Geometry check sheet. Reference: the model listing, model coordinates, mm. A direction names the side the tool comes from. Coordinates: 2 decimals unless noted, no trailing zeros. Write each loop counter-clockwise with the first axis right and the second up, starting at its lowest first coordinate (ties: lowest second). Pieces come first, ordered by that corner, then holes. Notation, with made-up numbers: M 23,-8 L 48,-8 A21 cw 48,30 Z; hole C 58.25,38.25 d1. An arc over 180 degrees is marked long. Write each question's results on one line, items separated by ' | '.
```python
from build123d import *

# Parameters (mm, degrees)
F0_R          = 3.75
F1_DEPTH      = 25
F2_W          = 29.9994934789
F2_H          = 9
F3_DEPTH      = 52
F5_DEPTH      = 25
F8_DEPTH      = 3.5
F8_DEPTH_BACK = 3.5


with BuildPart() as f1:
    # F0 (on Top) → F1 (new body)
    with BuildSketch(Plane.XY):
        with BuildLine():
            Line((0, 18.1232695296), (0, 0))
            Line((0, 0), (29.9994934789, 0))
            Line((29.9994934789, 0), (29.9994934789, 18))
            ThreePointArc((29.9994934789, 18), (15.061128764, 32.9998733692), (0, 18.1232695296))
        make_face()
        with Locations((14.9994934789, 18)):
            Circle(F0_R, mode=Mode.SUBTRACT)
    extrude(amount=F1_DEPTH)

    # F2 (on face) → F3 (join)
    with BuildSketch(Plane.XZ):
        with Locations((14.9997467394, 4.5)):
            Rectangle(F2_W, F2_H)
    extrude(amount=F3_DEPTH)

    # F4 (on face) → F5 (cut)
    with BuildSketch(Plane.XY.offset(9)):
        Polygon((20.9994934789, -52), (29.9994934789, -52), (29.9994934789, -43), align=None)
        Polygon((0, -43), (0, -52), (9, -52), align=None)
    extrude(amount=-F5_DEPTH, mode=Mode.SUBTRACT)

    # F7 (on mid) → F8 (join, two sides)
    with BuildSketch(Plane.YZ.offset(14.9997467394)) as f8_sk:
        Polygon((0, 9), (0, 25), (-52, 9), align=None)
    extrude(amount=F8_DEPTH)
    extrude(f8_sk.sketch, amount=-F8_DEPTH_BACK)


solid = f1.part
```
Q1. Mould release check, pull along Y, two halves, no side actions. Record for faces 4 (the flat face through (15, -52, 5)), 5 (the flat face through (0, -5, 7)), 6 (the cylindrical face through (14.19, 14.34, 12.32)): pulls with the +Y half, pulls with the -Y half, needs draft (parallel to the pull), parting line crosses it, or undercut.
Geometry check:
face 4: pulls with the -Y half | face 5: needs draft | face 6: undercut
Q2. Sectioned sample at A-A on z = 8.25. Record the cut outline in (x, y), and give its area (3 significant figures).
Geometry check:
outline: M 0,-43 L 9,-52 L 21,-52 L 30,-43 L 30,18 A15 ccw 0,18.12 Z; hole C 15,18 d7.5 | area: 2,330 mm2
Q3. Sectioned sample at C-C on y = -21. Record the cut outline in (x, z).
Geometry check:
outline: M 0,0 L 30,0 L 30,9 L 18.5,9 L 18.5,18.54 L 11.5,18.54 L 11.5,9 L 0,9 Z
Q4. Scan lines: probe 1 along X at (y, z) = (-11, 15.5); probe 2 along X at (y, z) = (15.5, 4.75); probe 3 along Z at (x, y) = (7, -29.5). Record each from-to range of solid material in increasing order.
Geometry check:
probe 1: x = 11.5 to 18.5 | probe 2: x = 0 to 12.2, 17.79 to 30 | probe 3: z = 0 to 9
Q5. Depth check by flat-ended pin: P1, Ø5, axis at y = -23, z = 18.5, coming from the -X side; P2, Ø4, axis at x = 4, z = 17, coming from the -Y side; P3, Ø8, axis at y = -14, z = 15.5, coming from the +X side. Enter the tip coordinate at first touch or a pass-through.
Geometry check:
P1: stops at x = 11.5 | P2: stops at y = 0 | P3: stops at x = 18.5
Q6. Sectioned sample at B-B on x = 3.25. Record the cut outline in (y, z), and give its area (3 significant figures).
Geometry check:
outline: M -46.25,0 L 27.32,0 L 27.32,25 L 0,25 L 0,9 L -46.25,9 Z | area: 1,100 mm2
Q7. Sectioned sample at D-D on z = 21.25. Record the cut outline in (x, y).
Geometry check:
outline: M 0,0 L 11.5,0 L 11.5,-12.19 L 18.5,-12.19 L 18.5,0 L 30,0 L 30,18 A15 ccw 0,18.12 Z; hole C 15,18 d7.5
Q8. Access from +Z, -Z, +X, -X, +Y, -Y to the whole of each face (thin tool, end or side, straight path). Record for faces 1 (the flat face through (26, -47, 5)), 2 (the flat face through (24, 0, 17)), 3 (the flat face through (11.5, -15, 14)).
Geometry check:
face 1: +Z, -Z, +X, -Y | face 2: +Z, +X, -Y | face 3: +Z, -X, -Y
